from build123d import *

# Parameters (mm, degrees)
SKETCH12_W          = 17
SKETCH12_H          = 41.5
SKETCH12_R          = 2
SKETCH12_R_2        = 4.05
SKETCH12_R_3        = 1.75
BOSS_EXTRUDE3_DEPTH = 10
SKETCH18_W          = 4.5
SKETCH18_H          = 7
SKETCH18_W_2        = 8
SKETCH18_H_2        = 1.5
BOSS_EXTRUDE4_DEPTH = 5
SKETCH23_R          = 2
CUT_EXTRUDE12_DEPTH = 2
CUT_EXTRUDE13_DEPTH = 46.948340558
CUT_EXTRUDE14_DEPTH = 9
FILLET4_R           = 0.5


with BuildPart() as part:
    # Sketch12 → Boss-Extrude3 (new body)
    with BuildSketch(Plane.XY):
        with Locations((-8.5, -20.75)):
            Rectangle(SKETCH12_W, SKETCH12_H)
        with Locations((-7, -9)):
            Circle(SKETCH12_R, mode=Mode.SUBTRACT)
        with Locations((-7, -21)):
            Circle(SKETCH12_R_2, mode=Mode.SUBTRACT)
        with Locations((-7, -33)):
            Circle(SKETCH12_R, mode=Mode.SUBTRACT)
        with Locations((-4, -28)):
            Circle(SKETCH12_R_3, mode=Mode.SUBTRACT)
    extrude(amount=BOSS_EXTRUDE3_DEPTH)

    # Sketch18 → Boss-Extrude4 (add)
    with BuildSketch(Plane.XY.offset(10)):
        with Locations((2.25, -14)):
            Rectangle(SKETCH18_W, SKETCH18_H)
        with Locations((2.25, -38)):
            Rectangle(SKETCH18_W, SKETCH18_H)
        with Locations((-13, 0.75)):
            Rectangle(SKETCH18_W_2, SKETCH18_H_2)
    extrude(amount=-BOSS_EXTRUDE4_DEPTH)

    # Sketch23 → Cut-Extrude12 (cut)
    with BuildSketch(Plane(origin=(0, 0, 0), x_dir=(-1, 0, 0), z_dir=(0, 0, -1))):
        with Locations((4, -28)):
            Circle(SKETCH23_R)
    extrude(amount=-CUT_EXTRUDE12_DEPTH, mode=Mode.SUBTRACT)

    # Sketch24 → Cut-Extrude13 (cut, through all)
    with BuildSketch(Plane(origin=(0, 0, 0), x_dir=(-1, 0, 0), z_dir=(0, 0, -1))):
        with BuildLine():
            Line((0, -34.5), (-4.5, -34.5))
            ThreePointArc((-4.5, -34.5), (-6, -33), (-4.5, -31.5))
            Line((-4.5, -31.5), (0, -31.5))
            ThreePointArc((0, -31.5), (1.5, -33), (0, -34.5))
        make_face()
        with BuildLine():
            Line((0, -20.5), (-4.5, -20.5))
            ThreePointArc((-4.5, -20.5), (-6, -19), (-4.5, -17.5))
            Line((-4.5, -17.5), (0, -17.5))
            ThreePointArc((0, -17.5), (1.5, -19), (0, -20.5))
        make_face()
        with BuildLine():
            Line((-4.5, -7.5), (0, -7.5))
            ThreePointArc((0, -7.5), (1.5, -9), (0, -10.5))
            Line((0, -10.5), (-4.5, -10.5))
            ThreePointArc((-4.5, -10.5), (-6, -9), (-4.5, -7.5))
        make_face()
        with BuildLine():
            Line((6, 0), (6, 1.5))
            ThreePointArc((6, 1.5), (7.5, 3), (9, 1.5))
            Line((9, 1.5), (9, 0))
            ThreePointArc((9, 0), (7.5, -1.5), (6, 0))
        make_face()
        with BuildLine():
            Line((19, 0), (19, 1.5))
            ThreePointArc((19, 1.5), (17.5, 3), (16, 1.5))
            Line((16, 1.5), (16, 0))
            ThreePointArc((16, 0), (17.5, -1.5), (19, 0))
        make_face()
    extrude(amount=-CUT_EXTRUDE13_DEPTH, mode=Mode.SUBTRACT)

    # Sketch25 → Cut-Extrude14 (cut)
    with BuildSketch(Plane(origin=(0, 0, 0), x_dir=(-1, 0, 0), z_dir=(0, 0, -1))):
        with BuildLine():
            Line((14.15, 1.5), (14.15, -6.35))
            ThreePointArc((14.15, -6.35), (12.5, -8), (10.85, -6.35))
            Line((10.85, -6.35), (10.85, 1.5))
            ThreePointArc((10.85, 1.5), (12.5, 3.15), (14.15, 1.5))
        make_face()
        with BuildLine():
            Line((-4.5, -12.35), (3.35, -12.35))
            ThreePointArc((3.35, -12.35), (5, -14), (3.35, -15.65))
            Line((3.35, -15.65), (-4.5, -15.65))
            ThreePointArc((-4.5, -15.65), (-6.15, -14), (-4.5, -12.35))
        make_face()
        with BuildLine():
            Line((-4.5, -36.35), (3.35, -36.35))
            ThreePointArc((3.35, -36.35), (5, -38), (3.35, -39.65))
            Line((3.35, -39.65), (-4.5, -39.65))
            ThreePointArc((-4.5, -39.65), (-6.15, -38), (-4.5, -36.35))
        make_face()
    extrude(amount=-CUT_EXTRUDE14_DEPTH, mode=Mode.SUBTRACT)

    # Fillet4
    fillet4_edges = [part.edges().sort_by_distance(p)[0] for p in [
        (4.5, -41.5, 7.5),
        (4.5, -10.5, 7.5),
        (4.5, -34.5, 7.5),
        (4.5, -17.5, 7.5),
        (-17, -41.5, 5),
        (0, 0, 5),
        (-9, 1.5, 7.5),
        (-16, 1.5, 7.5),
        (-14.15, 1.5, 7),
        (-10.85, 1.5, 7),
        (4.5, -36.35, 7),
        (4.5, -39.65, 7),
        (4.5, -15.65, 7),
        (4.5, -12.35, 7),
    ]]
    fillet(fillet4_edges, radius=FILLET4_R)


solid = part.part
Work out the finished part from the listing and answer in its coordinate system (mm). A direction names the side the tool comes from. Give positions to 0.01 mm unless a question says otherwise; leave off trailing zeros. Write each loop counter-clockwise with the first axis right and the second up, starting at its lowest first coordinate (ties: lowest second). Pieces come first, ordered by that corner, then holes. Notation, with made-up numbers: (6, 59.5) - (32, 59.5) arc R10 cw to (32, 63.5) - close; hole circle Ø1 at (56, 48). An arc over 180 degrees is marked (long way). One line per item, written item: value. Start each with the question number.
1. For faces 4 (the flat face through (-10, 0, 2)), 5 (the flat face through (0, -26, 5)), 6 (the flat face through (-1, -15.65, 5)), 7 (the cylindrical face through (-4, -30, 1)), determine the directions among +Z, -Z, +X, -X, +Y, -Y from which every point of the face is accessible in a straight line to the end or side of a thin tool.
2. For a pull along Y with two mould halves and no side action, classify faces 1 (the flat face through (2, -10.5, 8)), 2 (the flat face through (0, -17, 2)), 3 (the cylindrical face through (-7.878, -24.954, 4.93)) as +Y half, -Y half, draft (parallel to the pull), parting line (faces both ways), or undercut.
3. Consider probe 1 along Y at (x, z) = (-7, 3.5); probe 2 along Y at (x, z) = (0.5, 8.75); probe 3 along Y at (x, z) = (-4, 0.55). Determine where each line is inside the solid, lowest interval first.
4. Find section D-D (y = -9). Write down the section's boundary in (x, z).
5. Find section B-B (x = 2.25). Write down the section's boundary in (y, z).
6. Find section A-A (y = -28). Write down the section's boundary in (x, z).
7. Find section C-C (z = 1). State how many separate pieces and enclosed holes the cut face has, then the cut area to 3 significant figures.
8. Given pin 1 (0.6 mm diameter, centred on y = -11.5, z = 1.5, fed in from +X); pin 2 (2 mm diameter, centred on x = 2, z = 8, fed in from +Y); pin 3 (2 mm diameter, centred on x = 0, z = 6, fed in from +Y), each flat-ended and moving along its own axis, determine where each tip first touches the part or whether it passes through.
Geometry results:
1. face 4: -Z, +X, -X, +Y
1. face 5: +Z, -Z, +X
1. face 6: -Z, +X
1. face 7: -Z
2. face 1: +Y half
2. face 2: draft
2. face 3: undercut
3. probe 1: -41.5 to -35, -31 to -25.05, -16.95 to -11, -7 to -1.41
3. probe 2: -41.5 to -39.65, -36.35 to -34.5, -17.5 to -15.65, -12.35 to -10.5
3. probe 3: -41.5 to -39.52, -36.48 to -30, -26 to -23.72, -18.28 to -15.52, -12.48 to 0
4. outline: (-17, 0) - (-9, 0) - (-9, 10) - (-17, 10) - close; (-5, 0) - (-1.5, 0) - (-1.5, 10) - (-5, 10) - close
5. outline: (-41.5, 5) - (-39.65, 5) - (-39.65, 9) - (-36.35, 9) - (-36.35, 5) - (-34.5, 5) - (-34.5, 10) - (-41.5, 10) - close; (-17.5, 5) - (-15.65, 5) - (-15.65, 9) - (-12.35, 9) - (-12.35, 5) - (-10.5, 5) - (-10.5, 10) - (-17.5, 10) - close
6. outline: (-17, 0) - (-6, 0) - (-6, 2) - (-5.75, 2) - (-5.75, 10) - (-17, 10) - close; (-2.25, 2) - (-2, 2) - (-2, 0) - (0, 0) - (0, 10) - (-2.25, 10) - close
7. separate pieces: 1
7. enclosed holes: 4
7. area: 545 mm2
8. pin 1: x = 0
8. pin 2: y = -10.5
8. pin 3: y = 0
